Geometry check sheet. Reference: drawing and pictorial views, mm from the part's lowest x, y, z. A direction names the side the tool comes from. Give positions to 0.01 mm unless a question says otherwise; leave off trailing zeros. Order: outer loops, then holes, each group sorted by start corner. A loop starts at its lowest first (then second) coordinate and runs counter-clockwise, first axis right, second up. Notation, with made-up numbers: M -30.5,-31 L 18.5,-31 A20 cw 18.5,-26 Z; hole C 77.5,-23.5 d1. An arc over 180 degrees is marked long. Answer as CSV lines item,"result".
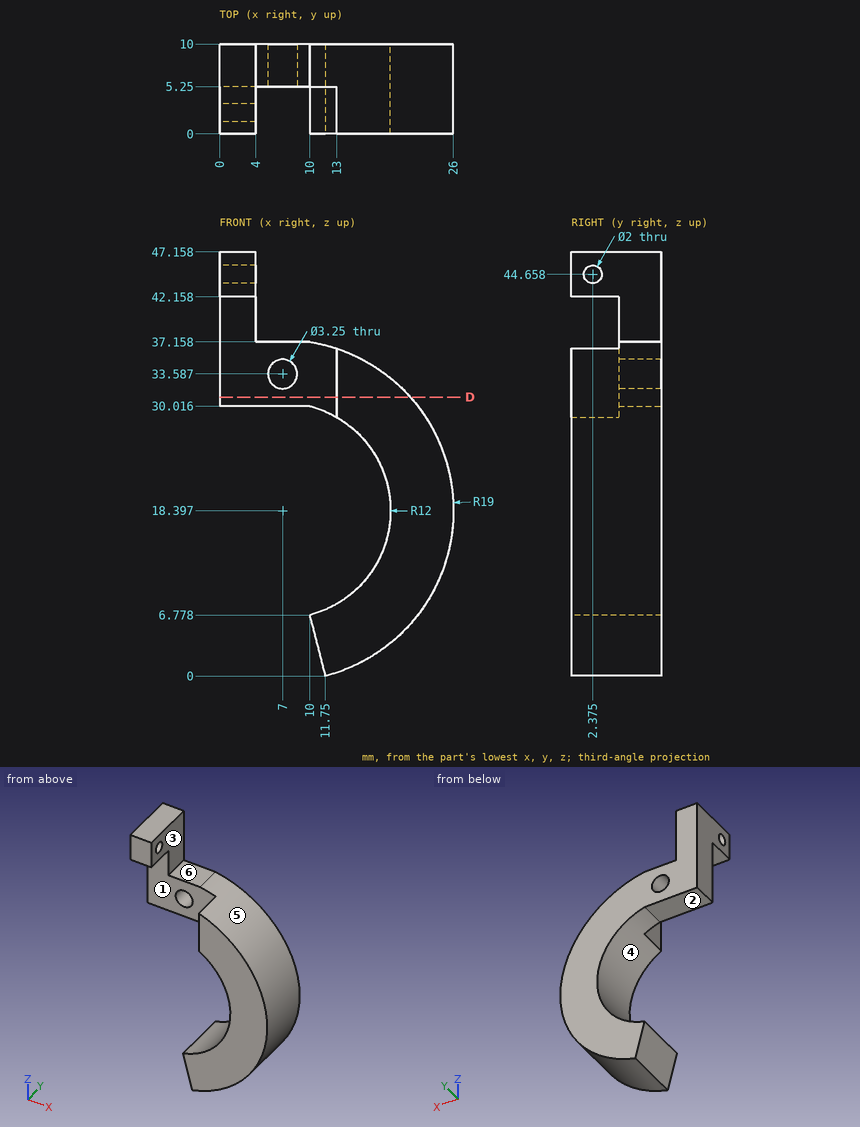
(1) Section check D-D on z = 31. Enter the section's corners in (x, y), then the cut area to 3 significant figures.
The answers:
outline,"M 0,5.25 L 13,5.25 L 13,0 L 21.22,0 L 21.22,10 L 0,10 Z"
area,"144 mm2"
(2) Gauge pin test, flat ends, axial feed: P1, Ø3.5, axis at x = 7, z = 33.587, coming from the -Y side; P2, Ø2, axis at x = 1, y = 2, coming from the -Z side; P3, Ø1.4, axis at x = 8.5, y = 7, coming from the +Z side. Record the tip position at first contact, or that the pin passes through.
The answers:
P1,"stops at y = 5.25"
P2,"stops at z = 42.16"
P3,"stops at z = 37.16"
(3) Draft check along Z on the marked faces 4, 5 and 6. Enter one of: +Z half, -Z half, draft (parallel to the pull), parting line (faces both ways), or undercut.
The answers:
face 4,"undercut"
face 5,"parting line"
face 6,"+Z half"
(4) Tool access check on the marked faces 1, 2 and 3. Record the directions out of +Z, -Z, +X, -X, +Y, -Y that give a thin tool (end or side, any length) a straight path to the whole face; none if there is none.
The answers:
face 1,"-X, -Y"
face 2,"-Z, -X, +Y, -Y"
face 3,"+Z, +X, +Y, -Y"
(5) Material ranges on line 1 (Z direction, x = 3, y = 2.5); line 2 (Z direction, x = 7, y = 6.95) (1 decimal); line 3 (X direction, y = 7, z = 33.5) (1 decimal), recorded low to high.
The answers:
line 1,"z = 42.16 to 43.67, 45.65 to 47.16"
line 2,"z = 30 to 32, 35.2 to 37.2"
line 3,"x = 0 to 5.4, 8.6 to 18.5"
